Verification items for the finished model (mm, model axes). Face numbers are marked on the shaded views. A direction names the side the tool comes from. Give positions to 0.01 mm unless a question says otherwise; leave off trailing zeros. Loops run counter-clockwise (first coordinate to the right, second up) from the corner with the lowest first, then second, coordinate; pieces in that order, holes last. Notation, with made-up numbers: (8, -21) - (50, -21) arc R9 cw to (50, -5) - close; hole circle Ø2 at (35.5, 52). An arc over 180 degrees is marked (long way). Put each result on its own line as item: value. Start each with the question number.
Autodesk Inventor part; units mm, degrees
ref_plane "YZ Plane" through (0, 0, 0) normal (1, 0, 0) x (0, 1, 0)
ref_plane "XZ Plane" through (0, 0, 0) normal (0, 1, 0) x (-1, 0, 0)
ref_plane "XY Plane" through (0, 0, 0) normal (0, 0, 1) x (1, 0, 0)
sketch "Esboço1" plane through (0, 0, 0) normal (0, 1, 0) x (-1, 0, 0)
  arc A0 (1, 1.118) -> (1, -1.118) centre (0, 0) ccw
  line L0 (1, 1.118) -> (1, -1.118)
  line L1 (0, 0) -> (-1.5, 0) construction
  line L2 (1.2, -1.2042) -> (1.2, 1.2042) construction
  arc A1 (1.2, 1.2042) -> (1.2, -1.2042) centre (0, 0) ccw construction
  circle A2 centre (0, 0) radius 3
  point P0 (1, 0)
  dimension "d0" = 3
  dimension "d1" = 2.5
  dimension "d2" = 0.2
  dimension "d3" = 6
extrude "Extrusão1" add sketch "Esboço1" along normal blind 4
sketch "Esboço2" plane through (0, 4, 0) normal (0, 1, 0) x (1, 0, 0)
  line L0 (0, 0) -> (-5, 0) construction
  line L1 (-5, 0) -> (-5, 0.25)
  line L2 (-5, 0.25) -> (-4.5, 0.5387)
  line L3 (-4.5, 0.5387) -> (-2.8873, 0.5387)
  line L4 (-5, 0) -> (-5, -0.25)
  line L5 (-5, -0.25) -> (-4.5, -0.5387)
  line L6 (-4.5, -0.5387) -> (-2.8873, -0.5387)
  line L7 (-4.3301, -2.5) -> (-4.4551, -2.2835)
  line L8 (-4.4551, -2.2835) -> (-4.1665, -1.7835)
  line L9 (-4.1665, -1.7835) -> (-2.7698, -0.9771)
  line L10 (-4.3301, -2.5) -> (-4.2051, -2.7165)
  line L11 (-4.2051, -2.7165) -> (-3.6278, -2.7165)
  line L12 (-3.6278, -2.7165) -> (-2.2311, -1.9102)
  line L13 (-2.5, -4.3301) -> (-2.7165, -4.2051)
  line L14 (-2.7165, -4.2051) -> (-2.7165, -3.6278)
  line L15 (-2.7165, -3.6278) -> (-1.9102, -2.2311)
  line L16 (-2.5, -4.3301) -> (-2.2835, -4.4551)
  line L17 (-2.2835, -4.4551) -> (-1.7835, -4.1665)
  line L18 (-1.7835, -4.1665) -> (-0.9771, -2.7698)
  line L19 (0, -5) -> (-0.25, -5)
  line L20 (-0.25, -5) -> (-0.5387, -4.5)
  line L21 (-0.5387, -4.5) -> (-0.5387, -2.8873)
  line L22 (0, -5) -> (0.25, -5)
  line L23 (0.25, -5) -> (0.5387, -4.5)
  line L24 (0.5387, -4.5) -> (0.5387, -2.8873)
  line L25 (2.5, -4.3301) -> (2.2835, -4.4551)
  line L26 (2.2835, -4.4551) -> (1.7835, -4.1665)
  line L27 (1.7835, -4.1665) -> (0.9771, -2.7698)
  line L28 (2.5, -4.3301) -> (2.7165, -4.2051)
  line L29 (2.7165, -4.2051) -> (2.7165, -3.6278)
  line L30 (2.7165, -3.6278) -> (1.9102, -2.2311)
  line L31 (4.3301, -2.5) -> (4.2051, -2.7165)
  line L32 (4.2051, -2.7165) -> (3.6278, -2.7165)
  line L33 (3.6278, -2.7165) -> (2.2311, -1.9102)
  line L34 (4.3301, -2.5) -> (4.4551, -2.2835)
  line L35 (4.4551, -2.2835) -> (4.1665, -1.7835)
  line L36 (4.1665, -1.7835) -> (2.7698, -0.9771)
  line L37 (5, 0) -> (5, -0.25)
  line L38 (5, -0.25) -> (4.5, -0.5387)
  line L39 (4.5, -0.5387) -> (2.8873, -0.5387)
  line L40 (5, 0) -> (5, 0.25)
  line L41 (5, 0.25) -> (4.5, 0.5387)
  line L42 (4.5, 0.5387) -> (2.8873, 0.5387)
  line L43 (4.3301, 2.5) -> (4.4551, 2.2835)
  line L44 (4.4551, 2.2835) -> (4.1665, 1.7835)
  line L45 (4.1665, 1.7835) -> (2.7698, 0.9771)
  line L46 (4.3301, 2.5) -> (4.2051, 2.7165)
  line L47 (4.2051, 2.7165) -> (3.6278, 2.7165)
  line L48 (3.6278, 2.7165) -> (2.2311, 1.9102)
  line L49 (2.5, 4.3301) -> (2.7165, 4.2051)
  line L50 (2.7165, 4.2051) -> (2.7165, 3.6278)
  line L51 (2.7165, 3.6278) -> (1.9102, 2.2311)
  line L52 (2.5, 4.3301) -> (2.2835, 4.4551)
  line L53 (2.2835, 4.4551) -> (1.7835, 4.1665)
  line L54 (1.7835, 4.1665) -> (0.9771, 2.7698)
  line L55 (0, 5) -> (0.25, 5)
  line L56 (0.25, 5) -> (0.5387, 4.5)
  line L57 (0.5387, 4.5) -> (0.5387, 2.8873)
  line L58 (0, 5) -> (-0.25, 5)
  line L59 (-0.25, 5) -> (-0.5387, 4.5)
  line L60 (-0.5387, 4.5) -> (-0.5387, 2.8873)
  line L61 (-2.5, 4.3301) -> (-2.2835, 4.4551)
  line L62 (-2.2835, 4.4551) -> (-1.7835, 4.1665)
  line L63 (-1.7835, 4.1665) -> (-0.9771, 2.7698)
  line L64 (-2.5, 4.3301) -> (-2.7165, 4.2051)
  line L65 (-2.7165, 4.2051) -> (-2.7165, 3.6278)
  line L66 (-2.7165, 3.6278) -> (-1.9102, 2.2311)
  line L67 (-4.3301, 2.5) -> (-4.2051, 2.7165)
  line L68 (-4.2051, 2.7165) -> (-3.6278, 2.7165)
  line L69 (-3.6278, 2.7165) -> (-2.2311, 1.9102)
  line L70 (-4.3301, 2.5) -> (-4.4551, 2.2835)
  line L71 (-4.4551, 2.2835) -> (-4.1665, 1.7835)
  line L72 (-4.1665, 1.7835) -> (-2.7698, 0.9771)
  circle A0 centre (0, 0) radius 3
  point P0 (-1.0091, -2.8252)
  point P1 (-1.9421, -2.2865)
  point P2 (-2.2865, -1.9421)
  point P3 (-2.8252, -1.0091)
  point P4 (-2.9512, -0.5387)
  point P5 (-2.9512, 0.5387)
  point P6 (-2.8252, 1.0091)
  point P7 (-2.2865, 1.9421)
  point P8 (-1.9421, 2.2865)
  point P9 (-1.0091, 2.8252)
  point P10 (-0.5387, 2.9512)
  point P11 (0.5387, 2.9512)
  point P12 (1.0091, 2.8252)
  point P13 (1.9421, 2.2865)
  point P14 (2.2865, 1.9421)
  point P15 (2.8252, 1.0091)
  point P16 (2.9512, 0.5387)
  point P17 (2.9512, -0.5387)
  point P18 (2.8252, -1.0091)
  point P19 (2.2865, -1.9421)
  point P20 (1.9421, -2.2865)
  point P21 (1.0091, -2.8252)
  point P22 (0.5387, -2.9512)
  point P23 (-0.5387, -2.9512)
  dimension "d15" = 6
  dimension "d6" = 5
  dimension "d7" = 0.25
  dimension "d9" = 60
  dimension "d10" = 0.5
  dimension "d13" = 360
extrude "Extrusão2" add sketch "Esboço2" against normal blind 4 contours L1 L2 L3 A0 L6 L5 L4 | L72 L71 L70 L67 L68 L69 A0 | A0 L12 L11 L10 L7 L8 L9 | L66 L65 L64 L61 L62 L63 A0 | A0 L18 L17 L16 L13 L14 L15 | L60 L59 L58 L55 L56 L57 A0 | A0 L24 L23 L22 L19 L20 L21 | L54 L53 L52 L49 L50 L51 A0 | A0 L30 L29 L28 L25 L26 L27 | L48 L47 L46 L43 L44 L45 A0 | A0 L36 L35 L34 L31 L32 L33 | L42 L41 L40 L37 L38 L39 A0
properties part number "Gear"
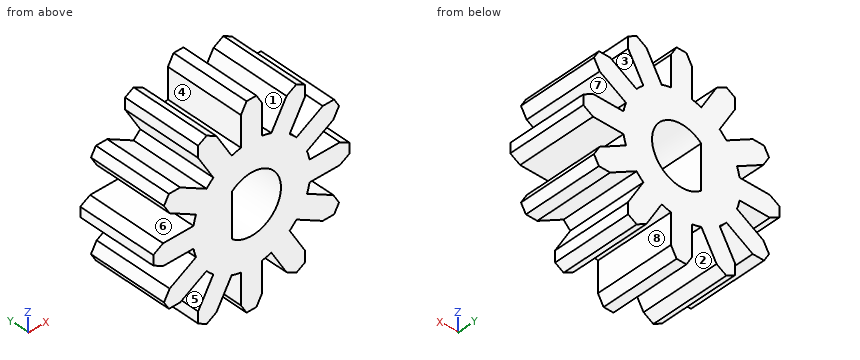
1) Section check A-A, the plane x = 0. Enter the section's corners in (y, z), plus the area to 3 significant figures.
2) Section check B-B, the plane z = 0. Enter the section's corners in (x, y).
3) Draft check along Z on the marked faces 1, 2, 3 and 4. Enter one of: pulls with the +Z half, pulls with the -Z half, needs draft (parallel to the pull), parting line crosses it, or undercut.
4) Depth check by flat-ended pin: P1, Ø2, axis at x = -3.5, y = 1, coming from the -Z side; P2, Ø2, axis at y = 0.5, z = -3.5, coming from the +X side; P3, Ø1.7, axis at x = -3.5, y = 1.5, coming from the +Z side. Enter the tip coordinate at first touch or a pass-through.
5) Scan lines: line 1 along Z through (x, y) = (0, 3); line 2 along X through (y, z) = (1.8, 0); line 3 along X through (y, z) = (2.65, 2.25). Record each from-to range of solid material in increasing order. Write a range as from..to.
6) Section check C-C, the plane x = -2.5. Enter the section's corners in (y, z), plus the area to 3 significant figures.
7) Set-up check for the marked faces 5, 6, 7 and 8: record each of +Z, -Z, +X, -X, +Y, -Y from which the full face is reachable in a straight line by a thin tool's end or side.
Results are:
1. outline: (0, -5) - (4, -5) - (4, -1.5) - (0, -1.5) - close; (0, 1.5) - (4, 1.5) - (4, 5) - (0, 5) - close
1. area: 28.0 mm2
2. outline: (-5, 0) - (-1, 0) - (-1, 4) - (-5, 4) - close; (1.5, 0) - (5, 0) - (5, 4) - (1.5, 4) - close
3. face 1: pulls with the +Z half
3. face 2: pulls with the -Z half
3. face 3: undercut
3. face 4: needs draft
4. P1: stops at z = -4.33
4. P2: stops at x = 4.33
4. P3: stops at z = 4.24
5. line 1: z = -5..-1.5, 1.5..5
5. line 2: x = -5..-1, 1.5..5
5. line 3: x = -4.44..-2.82, -1.98..1.98, 2.82..4.44
6. outline: (0, -4.33) - (4, -4.33) - (4, -3.25) - (0, -3.25) - close; (0, -2.07) - (4, -2.07) - (4, 2.07) - (0, 2.07) - close; (0, 3.25) - (4, 3.25) - (4, 4.33) - (0, 4.33) - close
6. area: 25.1 mm2
7. face 5: +Y, -Y
7. face 6: -X, +Y, -Y
7. face 7: +X, +Y, -Y
7. face 8: -Z, +Y, -Y
